Could you check a few things on this model? Use its own coordinates, in mm. Round coordinates to 2 decimals unless told otherwise and drop trailing zeros. Loops run counter-clockwise (first coordinate to the right, second up) from the corner with the lowest first, then second, coordinate; pieces in that order, holes last. Notation, with made-up numbers: M 73.5,33 L 81.5,33 A4 cw 81.5,39 Z; hole C 0.5,73.25 d11. An arc over 180 degrees is marked long. One line per item, written item: value. Start each with the question number.
Q1. Imagine slicing it at A-A (x = -5). Please give me the cut outline in (y, z), then the cut area to 3 significant figures.
Q2. Imagine slicing it at B-B (z = -13). Please give me the cut outline in (x, y), then the cut area to 3 significant figures.
Q3. Imagine slicing it at D-D (z = 14.85). Please give me the cut outline in (x, y).
Q4. I'm going to push a flat-ended pin straight in: pin 1 Ø1.5 at (x, z) = (-8, 9) entering from +Y. Where does the tip first touch, or does it pass through?
Q5. Please list where these lines run through material, in increasing order: line 1 along X through (y, z) = (0.65, -34.65); line 2 along X through (y, z) = (2.6, -22); line 3 along Z through (x, y) = (8, 1.45).
Q6. Imagine slicing it at C-C (y = 0.5). Please give me the cut outline in (x, z).
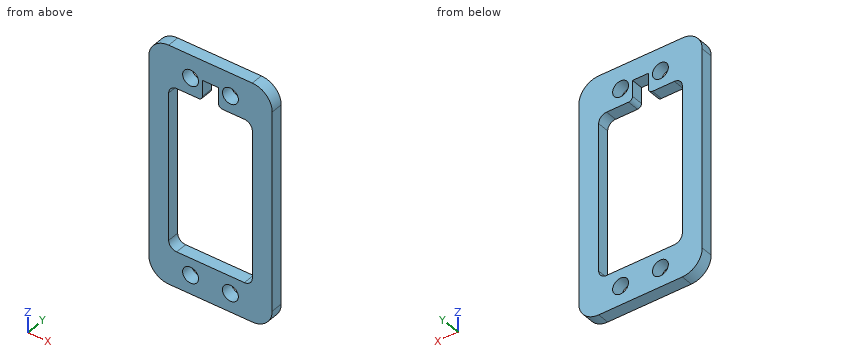
from build123d import *

# Parameters (mm, degrees)
SKETCH1_R           = 2
BOSS_EXTRUDE1_DEPTH = 3


with BuildPart() as part:
    # Sketch1 → Boss-Extrude1 (new body)
    with BuildSketch(Plane(origin=(0, 0, 0), x_dir=(1, 0, 0), z_dir=(0, 1, 0))):
        with BuildLine():
            ThreePointArc((-15.5, 34.4), (-14.035533906, 37.935533906), (-10.5, 39.4))
            Line((-10.5, 39.4), (10.5, 39.4))
            ThreePointArc((10.5, 39.4), (14.035533906, 37.935533906), (15.5, 34.4))
            Line((15.5, 34.4), (15.5, -15.6))
            ThreePointArc((15.5, -15.6), (14.035533906, -19.135533906), (10.5, -20.6))
            Line((10.5, -20.6), (-10.5, -20.6))
            ThreePointArc((-10.5, -20.6), (-14.035533906, -19.135533906), (-15.5, -15.6))
            Line((-15.5, -15.6), (-15.5, 34.4))
        make_face()
        with Locations(Location((5, -14.85, 0), (0, 0, 270))):
            Circle(SKETCH1_R, mode=Mode.SUBTRACT)
        with Locations(Location((-5, -14.85, 0), (0, 0, 270))):
            Circle(SKETCH1_R, mode=Mode.SUBTRACT)
        with Locations(Location((5, 34.65, 0), (0, 0, 270))):
            Circle(SKETCH1_R, mode=Mode.SUBTRACT)
        with Locations(Location((-5, 34.65, 0), (0, 0, 270))):
            Circle(SKETCH1_R, mode=Mode.SUBTRACT)
        with BuildLine():
            ThreePointArc((-3, -10.6), (-2.292893219, -10.892893219), (-2, -11.6))
            Line((-2, -11.6), (-2, -15.6))
            Line((-2, -15.6), (2, -15.6))
            Line((2, -15.6), (2, -11.6))
            ThreePointArc((2, -11.6), (2.292893219, -10.892893219), (3, -10.6))
            Line((3, -10.6), (8.5, -10.6))
            ThreePointArc((8.5, -10.6), (9.914213562, -10.014213562), (10.5, -8.6))
            Line((10.5, -8.6), (10.5, 28.4))
            ThreePointArc((10.5, 28.4), (9.914213562, 29.814213562), (8.5, 30.4))
            Line((8.5, 30.4), (-8.5, 30.4))
            ThreePointArc((-8.5, 30.4), (-9.914213562, 29.814213562), (-10.5, 28.4))
            Line((-10.5, 28.4), (-10.5, -8.6))
            ThreePointArc((-10.5, -8.6), (-9.914213562, -10.014213562), (-8.5, -10.6))
            Line((-8.5, -10.6), (-3, -10.6))
        make_face(mode=Mode.SUBTRACT)
    extrude(amount=BOSS_EXTRUDE1_DEPTH)


solid = part.part
Report:
1. outline: M 0,-39.4 L 3,-39.4 L 3,-36.65 L 0,-36.65 Z; M 0,-32.65 L 3,-32.65 L 3,-30.4 L 0,-30.4 Z; M 0,10.6 L 3,10.6 L 3,12.85 L 0,12.85 Z; M 0,16.85 L 3,16.85 L 3,20.6 L 0,20.6 Z
1. area: 33.0 mm²
2. outline: M -15.5,0 L -10.5,0 L -10.5,3 L -15.5,3 Z; M 10.5,0 L 15.5,0 L 15.5,3 L 10.5,3 Z
2. area: 30.0 mm²
3. outline: M -15.5,0 L -7,0 L -7,3 L -15.5,3 Z; M -3,0 L -2,0 L -2,3 L -3,3 Z; M 2,0 L 3,0 L 3,3 L 2,3 Z; M 7,0 L 15.5,0 L 15.5,3 L 7,3 Z
4. pin 1: passes through
5. line 1: x = -15.49 to -7, -3 to 3, 7 to 15.49
5. line 2: x = -15.5 to -10.5, 10.5 to 15.5
5. line 3: z = -39.4 to -30.4, 10.6 to 20.6
6. outline: M -15.5,-34.4 A5 ccw -10.5,-39.4 L 10.5,-39.4 A5 ccw 15.5,-34.4 L 15.5,15.6 A5 ccw 10.5,20.6 L -10.5,20.6 A5 ccw -15.5,15.6 Z; hole M -10.5,-28.4 A2 ccw -8.5,-30.4 L 8.5,-30.4 A2 ccw 10.5,-28.4 L 10.5,8.6 A2 ccw 8.5,10.6 L 3,10.6 A1 cw 2,11.6 L 2,15.6 L -2,15.6 L -2,11.6 A1 cw -3,10.6 L -8.5,10.6 A2 ccw -10.5,8.6 Z; hole C -5,-34.65 d4; hole C -5,14.85 d4; hole C 5,-34.65 d4; hole C 5,14.85 d4
